The model under review builds one solid part; all positions refer to its coordinate system, in mm. Face numbers are marked on the shaded views. A direction names the side the tool comes from. Round coordinates to 2 decimals unless told otherwise and drop trailing zeros. Order: outer loops, then holes, each group sorted by start corner. A loop starts at its lowest first (then second) coordinate and runs counter-clockwise, first axis right, second up. Notation, with made-up numbers: M -4.5,31.5 L 13.5,31.5 A11 ccw 13.5,48.5 Z; hole C 15.5,59.5 d8. An arc over 180 degrees is marked long. Answer as a JSON object with one key per item and string values. Group by question number.
1) Insertion check: pin 1 Ø4 at (x, y) = (-29, -19) entering from -Z; pin 2 Ø1.5 at (y, z) = (0.5, -19.5) entering from -X; pin 3 Ø5 at (x, y) = (-25.5, 4) entering from -Z. Each pin has a flat end and moves straight along its axis. Give the tip position at first contact, or say it passes through.
2) The part is to be moulded in two halves that separate along Y. For the marked faces 1, 2 and 3, say which applies: +Y half, -Y half, draft (parallel to the pull), parting line (faces both ways), or undercut.
3) Consider section B-B, the plane x = 17.5. Write out the cut boundary in (y, z).
4) Consider section A-A, the plane z = 29. Write out the cut boundary in (x, y).
5) Consider section D-D, the plane z = -24. Write out the cut boundary in (x, y).
6) To check wall thickness, follow line 1 (Y direction, x = 17.5, z = 13); line 2 (X direction, y = -19, z = 8.5); line 3 (Y direction, x = 19, z = -27). State the ranges of each line that lie inside material, in increasing order.
7) Consider section C-C, the plane y = 17. Write out the cut boundary in (x, z).
8) For the marked faces 4 and 5, list the 3-axis set-ups (+Z, -Z, +X, -X, +Y, -Y) from which the entire face can be reached by the end or side of a thin tool; tool diameter is ignored.
```python
from build123d import *

# Parameters (mm, degrees)
F1_DEPTH = 35
F0_W     = 5.1
F0_H     = 5.1
F2_DEPTH = 12.5
F4_DEPTH = 22.5
F5_R     = 5
F6_R     = 1
F7_R     = 7
F7_R_2   = 15
F8_DEPTH = 65


with BuildPart() as f1:
    # F0 (on Top) → F1 (new body, symmetric)
    with BuildSketch(Plane.XY):
        Polygon((-11.9, 27.5), (-27.5, 27.5), (-27.5, 12.3), (-27.5, -11.9), (-27.5, -27.5), (-10.1801488287, -27.5), (10.1801488287, -27.5), (27.5, -27.5), (27.5, -10.1801488287), (27.5, 10.1801488287), (27.5, 27.5), (12.3, 27.5), align=None)
    extrude(amount=F1_DEPTH, both=True)

    # F0 (on Top) → F2 (join, symmetric)
    with BuildSketch(Plane.XY):
        Polygon((-27.5, 12.3), (-27.5, 27.5), (-32.6, 27.5), (-32.6, 10.4437518052), align=None)
        Polygon((-27.5, -27.5), (-27.5, -11.9), (-32.6, -10.0437518052), (-32.6, -27.5), align=None)
        Polygon((-27.5, 32.6), (-27.5, 27.5), (-11.9, 27.5), (-10.0437518052, 32.6), align=None)
        Polygon((10.4437518052, 32.6), (12.3, 27.5), (27.5, 27.5), (27.5, 32.6), align=None)
        Polygon((10.1801488287, -27.5), (-10.1801488287, -27.5), (-12, -32.5), (12, -32.5), align=None)
        Polygon((32.5, 12), (27.5, 10.1801488287), (27.5, -10.1801488287), (32.5, -12), align=None)
        with Locations((-30.05, 30.05)):
            Rectangle(F0_W, F0_H)
    extrude(amount=F2_DEPTH, both=True)

    # F3 (on face) → F4 (join, through all)
    with BuildSketch(Plane(origin=(0, 0, -35), x_dir=(1, 0, 0), z_dir=(0, 0, -1))):
        Polygon((-27.5, 32.5), (-27.5, 27.5), (27.5, 27.5), (27.5, -27.5), (32.5, -27.5), (32.5, 32.5), align=None)
    extrude(amount=-F4_DEPTH)

    # F5
    f5_edges = [f1.edges().sort_by_distance(p)[0] for p in [
        (-32.6, 32.6, 0),
        (-27.5, 27.5, 23.75),
        (-27.5, 27.5, -23.75),
        (-32.6, -27.5, 0),
        (-27.5, -32.5, -23.75),
        (32.5, -32.5, -23.75),
        (27.5, -27.5, 11.25),
        (32.5, 27.5, -23.75),
        (27.5, 32.6, 0),
        (27.5, 27.5, 23.75),
        (32.5, -2.5, -35),
        (2.5, -32.5, -35),
        (-27.5, -2.5, -35),
        (2.5, 27.5, -35),
        (-27.5, -27.5, 23.75),
    ]]
    fillet(f5_edges, radius=F5_R)

    # F6
    f6_edges = [f1.edges().sort_by_distance(p)[0] for p in [
        (12, -32.5, 0),
        (-12, -32.5, 0),
        (32.5, -12, 0),
        (32.5, 12, 0),
        (10.443752, 32.6, 0),
        (-10.043752, 32.6, 0),
        (-32.6, 10.443752, 0),
        (-32.6, -10.043752, 0),
    ]]
    fillet(f6_edges, radius=F6_R)

    # F7 (on face) → F8 (cut)
    with BuildSketch(Plane.XY.offset(35)):
        with Locations((17.5, 17)):
            Circle(F7_R)
        with Locations((17.5, 0)):
            Circle(F7_R)
        with Locations((17.5, -17)):
            Circle(F7_R)
        with Locations((-17, 17)):
            Circle(F7_R)
        with Locations((0, 17)):
            Circle(F7_R)
        with Locations((-8.5, -9.5)):
            Circle(F7_R_2)
    extrude(amount=-F8_DEPTH, mode=Mode.SUBTRACT)


solid = f1.part
```
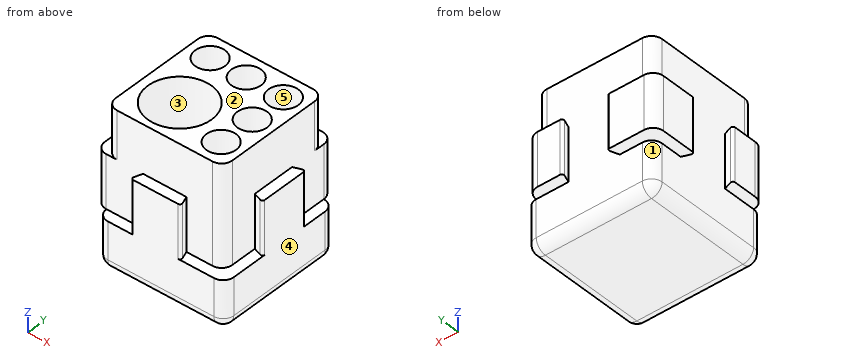
Results list:
{
 "1": {"pin 1": "z = -32.18", "pin 2": "x = -27.5", "pin 3": "z = -34.97"},
 "2": {"face 1": "+Y half", "face 2": "draft", "face 3": "undercut"},
 "3": {"outline": "M -32.5,-30 A5 ccw -27.5,-35 L 22.5,-35 A5 ccw 27.5,-30 L 27.5,-12.5 L 32.6,-12.5 L 32.6,12.5 L 27.5,12.5 L 27.5,35 L 24,35 L 24,-30 L 10,-30 L 10,35 L 7,35 L 7,-30 L -7,-30 L -7,35 L -10,35 L -10,-30 L -24,-30 L -24,35 L -27.5,35 L -27.5,-12.5 L -32.5,-12.5 Z"},
 "4": {"outline": "M -27.5,-22.5 A5 ccw -22.5,-27.5 L 22.5,-27.5 A5 ccw 27.5,-22.5 L 27.5,22.5 A5 ccw 22.5,27.5 L -22.5,27.5 A5 ccw -27.5,22.5 Z; hole C -17,17 d14; hole C -8.5,-9.5 d30; hole C 0,17 d14; hole C 17.5,-17 d14; hole C 17.5,0 d14; hole C 17.5,17 d14"},
 "5": {"outline": "M -27.5,-27.5 A5 ccw -22.5,-32.5 L 27.5,-32.5 A5 ccw 32.5,-27.5 L 32.5,22.5 A5 ccw 27.5,27.5 L -22.5,27.5 A5 ccw -27.5,22.5 Z; hole C -17,17 d14; hole C -8.5,-9.5 d30; hole C 0,17 d14; hole C 17.5,-17 d14; hole C 17.5,0 d14; hole C 17.5,17 d14"},
 "6": {"line 1": "-27.5 to -24, -10 to -7, 7 to 10, 24 to 27.5", "line 2": "-32.6 to -20.11, 3.11 to 10.79, 24.21 to 27.5", "line 3": "-32.5 to -23.84, -10.16 to -6.84, 6.84 to 10.16, 23.84 to 27.5"},
 "7": {"outline": "M -32.6,-12.5 L -27.5,-12.5 L -27.5,-30 A5 ccw -22.5,-35 L 27.5,-35 A5 ccw 32.5,-30 L 32.5,-12.5 L 27.5,-12.5 L 27.5,35 L 24.5,35 L 24.5,-30 L 10.5,-30 L 10.5,35 L 7,35 L 7,-30 L -7,-30 L -7,35 L -10,35 L -10,-30 L -24,-30 L -24,35 L -27.5,35 L -27.5,12.5 L -32.6,12.5 Z"},
 "8": {"face 4": "+Z, -Z, +X, +Y, -Y", "face 5": "+Z"}
}
